from build123d import *

# Parameters (mm, degrees)
ESQUISSE1_W                   = 460.2
ESQUISSE1_H                   = 60.2
BOSS_EXTRU_1_DEPTH            = 5
DIAM_TRE_DU_PER_AGE_1_0_1_1_D = 1
ENL_V_MAT_EXTRU_1_REACH       = 7


with BuildPart() as part:
    # Esquisse1 → Boss.-Extru.1 (new body)
    with BuildSketch(Plane.XY):
        with Locations((230, 30)):
            Rectangle(ESQUISSE1_W, ESQUISSE1_H)
    extrude(amount=BOSS_EXTRU_1_DEPTH)

    # Diamètre du perçage Ø1.0 (1)1 (through all)
    with Locations(Plane.XY.offset(5)):
        with Locations((5, 55), (5, 5), (455, 5), (455, 55)):
            Hole(DIAM_TRE_DU_PER_AGE_1_0_1_1_D / 2)

    # Esquisse4 → Enlèv. mat.-Extru.1 (cut, up to next)
    with BuildSketch(Plane.XY.offset(5), mode=Mode.PRIVATE) as enl_v_mat_extru_1_sk1:
        with BuildLine():
            Line((460.1, 10.1), (460.1, 49.9))
            Line((460.1, 49.9), (458.1, 49.9))
            ThreePointArc((458.1, 49.9), (451.099642866, 47.000357134), (448.2, 40))
            Line((448.2, 40), (448.2, 20))
            ThreePointArc((448.2, 20), (451.099642866, 12.999642866), (458.1, 10.1))
            Line((458.1, 10.1), (460.1, 10.1))
        make_face()
    enl_v_mat_extru_1_tool1 = extrude(enl_v_mat_extru_1_sk1.sketch, amount=-ENL_V_MAT_EXTRU_1_REACH, mode=Mode.PRIVATE) & part.part
    add(enl_v_mat_extru_1_tool1.solids().sort_by_distance((454.51443, 30, 5))[0], mode=Mode.SUBTRACT)


solid = part.part
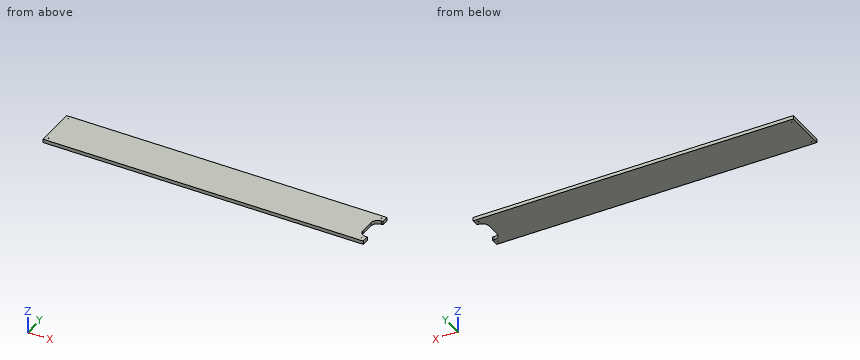
Can you work these out from the model? Positions are in its coordinate system, mm. Coordinates: 2 decimals unless noted, no trailing zeros. Order: outer loops, then holes, each group sorted by start corner. A loop starts at its lowest first (then second) coordinate and runs counter-clockwise, first axis right, second up. Notation, with made-up numbers: (3.5, -4.75) - (62.5, -4.75) arc R19 cw to (62.5, 23.25) - close; hole circle Ø10 at (65, -13). An arc over 180 degrees is marked (long way). Answer as a JSON object with one key per item and string values. Group by question number.
Q1. Imagine slicing it at A-A (z = 2.8). Please give me the cut outline in (x, y).
Q2. Will this pin go through, and if not, where does the flat tip stop? P1, Ø1.5, axis at y = 34, z = 3, coming from the +X side.
Q3. I need wall thicknesses on line 1 (X direction, y = 55, z = 2.9); line 2 (Y direction, x = 5, z = 3.15); line 3 (Y direction, x = 455, z = 1.6). Which ranges of each line are inside material? Lowest first, please. Write a range as from..to.
Q4. Imagine slicing it at B-B (y = 24). Please give me the cut outline in (x, z).
Determined:
{
 "1": {"outline": "(-0.1, -0.1) - (460.1, -0.1) - (460.1, 10.1) - (458.1, 10.1) arc R9.9 cw to (448.2, 20) - (448.2, 40) arc R9.9 cw to (458.1, 49.9) - (460.1, 49.9) - (460.1, 60.1) - (-0.1, 60.1) - close; hole circle Ø1 at (5, 5); hole circle Ø1 at (5, 55); hole circle Ø1 at (455, 5); hole circle Ø1 at (455, 55)"},
 "2": {"P1": "stops at x = 448.2"},
 "3": {"line 1": "x = -0.1..4.5, 5.5..454.5, 455.5..460.1", "line 2": "y = -0.1..4.5, 5.5..54.5, 55.5..60.1", "line 3": "y = -0.1..4.5, 5.5..10.6, 49.4..54.5, 55.5..60.1"},
 "4": {"outline": "(-0.1, 0) - (448.2, 0) - (448.2, 5) - (-0.1, 5) - close"}
}
